Part model, mm, in its own coordinate system. A direction names the side the tool comes from. Coordinates: 2 decimals unless noted, no trailing zeros. Order: outer loops, then holes, each group sorted by start corner. A loop starts at its lowest first (then second) coordinate and runs counter-clockwise, first axis right, second up. Notation, with made-up numbers: (19.25, 30.5) - (53.25, 30.5) arc R17 cw to (53.25, 37.5) - close; hole circle Ø3 at (6, 21). An arc over 180 degrees is marked (long way). Use a Markdown table: item, result. Add a question column.
1) Two-plate mould, pull along Y, no slides. Class faces 1 (the face through (22.59, -22.19, -12.5)), 2 (the face through (38, -25.1, 0)), 3 (the face through (-12.497, -0.275, 24.217)): +Y half, -Y half, draft (parallel to the pull), parting line (faces both ways), or undercut.
2) Saw through at B-B on y = 0. List the corners of the cut face in (x, z).
3) Saw through at D-D on x = -8. List the corners of the cut face in (y, z).
4) Saw through at A-A on x = 6. List the corners of the cut face in (y, z).
5) Tool access for faces 4 (the face through (16.3, 12.5, -23.4)), 5 (the face through (3, 0, -23)), 6 (the face through (38, 24.8, 0)), 7 (the face through (22, -22, 12.5)), 8 (the face through (25, 25, 12.5)): list every direction of +Z, -Z, +X, -X, +Y, -Y with a clear straight run to the whole face (end or side of a thin tool).
6) Drop flat-ended pins along their axis: P1, Ø12, axis at x = 28, y = 16.5, coming from the +Z side; P2, Ø5, axis at y = 13.5, z = 9, coming from the -X side; P3, Ø7.5, axis at x = 27.5, y = 19, coming from the -Z side; P4, Ø6.5, axis at x = 13, z = -21.5, coming from the -Y side. Give the stop position or say it passes through.
7) Saw through at C-C on z = 0. List the corners of the cut face in (x, y).
8) Wall check: L1, parallel to Y at x = 30.5, z = -11; L2, parallel to X at y = -8.5, z = -17; L3, parallel to Z at x = -4, y = 7.5. Give the ranges that are in metal, low to high. Write a range as [from, to].
```python
from build123d import *

# Parameters (mm, degrees)
EXTRUDE_5_DEPTH          = 25.4
EXTRUDE_5_DEPTH_BACK     = 25.7
CUT_EXTRUDE_1_DEPTH      = 23
CUT_EXTRUDE_1_DEPTH_BACK = 23
EXTRUDE_6_DEPTH          = 27.5
CUT_EXTRUDE_2_DEPTH      = 24.8
CUT_EXTRUDE_2_DEPTH_BACK = 25.1


with BuildPart() as part:
    # Эскиз5 → Бобышка-Вытянуть5 (new body, two sides)
    with BuildSketch(Plane.XY) as extrude_5_sk:
        with BuildLine():
            Line((0, 12.5), (22.75, 12.5))
            Line((22.75, 12.5), (22.75, -12.5))
            Line((22.75, -12.5), (0, -12.5))
            ThreePointArc((0, -12.5), (-12.5, 0), (0, 12.5))
        make_face()
    extrude(amount=EXTRUDE_5_DEPTH)
    extrude(extrude_5_sk.sketch, amount=-EXTRUDE_5_DEPTH_BACK)

    # Эскиз6 → Вырез-Вытянуть1 (cut, two sides)
    with BuildSketch(Plane.XY) as cut_extrude_1_sk:
        with BuildLine():
            Line((0, 12.5), (18.75, 12.5))
            Line((18.75, 12.5), (18.75, -12.5))
            Line((18.75, -12.5), (0, -12.5))
            ThreePointArc((0, -12.5), (-12.5, 0), (0, 12.5))
        make_face()
    extrude(amount=CUT_EXTRUDE_1_DEPTH, mode=Mode.SUBTRACT)
    extrude(cut_extrude_1_sk.sketch, amount=-CUT_EXTRUDE_1_DEPTH_BACK, mode=Mode.SUBTRACT)

    # Эскиз7 → Бобышка-Вытянуть6 (add, symmetric)
    with BuildSketch(Plane(origin=(0, 0, 0), x_dir=(1, 0, 0), z_dir=(0, 1, 0))):
        with BuildLine():
            Line((41.5, 12.5), (18.75, 12.5))
            Line((18.75, 12.5), (18.75, -12.5))
            Line((18.75, -12.5), (41.5, -12.5))
            ThreePointArc((41.5, -12.5), (54, 0), (41.5, 12.5))
        make_face()
    extrude(amount=EXTRUDE_6_DEPTH, both=True)

    # Эскиз8 → Вырез-Вытянуть2 (cut, two sides)
    with BuildSketch(Plane(origin=(0, 0, 0), x_dir=(1, 0, 0), z_dir=(0, 1, 0))) as cut_extrude_2_sk:
        with BuildLine():
            Line((41.5, 12.5), (22.75, 12.5))
            Line((22.75, 12.5), (22.75, -12.5))
            Line((22.75, -12.5), (41.5, -12.5))
            ThreePointArc((41.5, -12.5), (54, 0), (41.5, 12.5))
        make_face()
    extrude(amount=CUT_EXTRUDE_2_DEPTH, mode=Mode.SUBTRACT)
    extrude(cut_extrude_2_sk.sketch, amount=-CUT_EXTRUDE_2_DEPTH_BACK, mode=Mode.SUBTRACT)


solid = part.part
```
Results are:
| question | item | result |
|---|---|---|
| 1 | face 1 | draft |
| 1 | face 2 | undercut |
| 1 | face 3 | parting line |
| 2 | outline | (-12.5, -25.7) - (22.75, -25.7) - (22.75, 25.4) - (-12.5, 25.4) - (-12.5, 23) - (18.75, 23) - (18.75, -23) - (-12.5, -23) - close |
| 3 | outline | (-9.6, -25.7) - (9.6, -25.7) - (9.6, -23) - (-9.6, -23) - close; (-9.6, 23) - (9.6, 23) - (9.6, 25.4) - (-9.6, 25.4) - close |
| 4 | outline | (-12.5, -25.7) - (12.5, -25.7) - (12.5, -23) - (-12.5, -23) - close; (-12.5, 23) - (12.5, 23) - (12.5, 25.4) - (-12.5, 25.4) - close |
| 5 | face 4 | -Z, +X, -X, +Y |
| 5 | face 5 | -X, +Y, -Y |
| 5 | face 6 | +Z, -Z, +X |
| 5 | face 7 | +Z, +X, -X, -Y |
| 5 | face 8 | +Z, +X, -X, +Y |
| 6 | P1 | z = 12.5 |
| 6 | P2 | x = 18.75 |
| 6 | P3 | through |
| 6 | P4 | y = -12.5 |
| 7 | outline | (18.75, -27.5) - (54, -27.5) - (54, -25.1) - (22.75, -25.1) - (22.75, 24.8) - (54, 24.8) - (54, 27.5) - (18.75, 27.5) - close |
| 8 | L1 | [-27.5, -25.1], [24.8, 27.5] |
| 8 | L2 | [18.75, 22.75] |
| 8 | L3 | [-25.7, -23], [23, 25.4] |
